```python
from build123d import *

# Parameters (mm, degrees)
SKETCH_1_W               = 130
SKETCH_1_H               = 180
EXTRUDE_1_DEPTH          = 400
SKETCH_2_R               = 37.5
CUT_EXTRUDE_1_DEPTH      = 458.493169348
CUT_EXTRUDE_START        = -350
CUT_EXTRUDE_2_DEPTH      = 350
PATTERN_CIRCULAR_1_COUNT = 4
MIRROR_START             = -350
MIRROR_1_COPY_1_DEPTH    = 350
MIRROR_1_COPY_2_DEPTH    = 350
MIRROR_1_COPY_3_DEPTH    = 350


with BuildPart() as part:
    # Sketch 1 → Extrude 1 (new body)
    with BuildSketch(Plane.XY):
        with Locations((-65, 90)):
            Rectangle(SKETCH_1_W, SKETCH_1_H)
    extrude(amount=EXTRUDE_1_DEPTH)

    # Sketch 2 → Cut-Extrude 1 (cut, through all)
    with BuildSketch(Plane.XY.offset(400)):
        with Locations((-65, 132.5)):
            Circle(SKETCH_2_R)
        with Locations((-65, 47.5)):
            Circle(SKETCH_2_R)
    extrude(amount=-CUT_EXTRUDE_1_DEPTH, mode=Mode.SUBTRACT)

    # Sketch 4 → Cut-Extrude 2 (cut)
    with BuildSketch(Plane(origin=(0, 0, 0), x_dir=(-1, 0, 0), z_dir=(0, 0, -1)).offset(CUT_EXTRUDE_START)):
        with BuildLine():
            Line((86.25, 169.306079661), (83.75, 164.975952642))
            ThreePointArc((83.75, 164.975952642), (91.516504294, 159.016504294), (97.475952642, 151.25))
            Line((97.475952642, 151.25), (101.806079661, 153.75))
            ThreePointArc((101.806079661, 153.75), (95.0520382, 162.5520382), (86.25, 169.306079661))
        make_face()
    cut_extrude_2 = extrude(amount=CUT_EXTRUDE_2_DEPTH, mode=Mode.SUBTRACT)

    # Pattern Circular 1: Cut-Extrude 2 ×4 about axis
    pattern_circular_1_axis = Axis((-65, 132.5, 0), (0, 0, 1))
    for i in range(1, PATTERN_CIRCULAR_1_COUNT):
        add(cut_extrude_2.rotate(pattern_circular_1_axis, i * 360 / PATTERN_CIRCULAR_1_COUNT), mode=Mode.SUBTRACT)

    # Mirror 1: Cut-Extrude 2 across plane
    add(cut_extrude_2.mirror(Plane.ZX.offset(90)), mode=Mode.SUBTRACT)

    # Mirror 1 copy 1 sketch → Mirror 1 copy 1 (cut)
    with BuildSketch(Plane(origin=(67.5, -17.5, 0), x_dir=(0, 1, 0), z_dir=(0, 0, -1)).offset(MIRROR_START)):
        with BuildLine():
            Line((86.25, -169.306079661), (83.75, -164.975952642))
            ThreePointArc((83.75, -164.975952642), (91.516504294, -159.016504294), (97.475952642, -151.25))
            Line((97.475952642, -151.25), (101.806079661, -153.75))
            ThreePointArc((101.806079661, -153.75), (95.0520382, -162.5520382), (86.25, -169.306079661))
        make_face()
    extrude(amount=MIRROR_1_COPY_1_DEPTH, mode=Mode.SUBTRACT)

    # Mirror 1 copy 2 sketch → Mirror 1 copy 2 (cut)
    with BuildSketch(Plane(origin=(-130, -85, 0), x_dir=(1, 0, 0), z_dir=(0, 0, -1)).offset(MIRROR_START)):
        with BuildLine():
            Line((86.25, -169.306079661), (83.75, -164.975952642))
            ThreePointArc((83.75, -164.975952642), (91.516504294, -159.016504294), (97.475952642, -151.25))
            Line((97.475952642, -151.25), (101.806079661, -153.75))
            ThreePointArc((101.806079661, -153.75), (95.0520382, -162.5520382), (86.25, -169.306079661))
        make_face()
    extrude(amount=MIRROR_1_COPY_2_DEPTH, mode=Mode.SUBTRACT)

    # Mirror 1 copy 3 sketch → Mirror 1 copy 3 (cut)
    with BuildSketch(Plane(origin=(-197.5, 112.5, 0), x_dir=(0, -1, 0), z_dir=(0, 0, -1)).offset(MIRROR_START)):
        with BuildLine():
            Line((86.25, -169.306079661), (83.75, -164.975952642))
            ThreePointArc((83.75, -164.975952642), (91.516504294, -159.016504294), (97.475952642, -151.25))
            Line((97.475952642, -151.25), (101.806079661, -153.75))
            ThreePointArc((101.806079661, -153.75), (95.0520382, -162.5520382), (86.25, -169.306079661))
        make_face()
    extrude(amount=MIRROR_1_COPY_3_DEPTH, mode=Mode.SUBTRACT)


solid = part.part
```
The listing builds one solid part. Answer for the finished solid, in the listing's coordinates (mm). A direction names the side the tool comes from. Coordinates: 2 decimals unless noted, no trailing zeros. Write each loop counter-clockwise with the first axis right and the second up, starting at its lowest first coordinate (ties: lowest second). Pieces come first, ordered by that corner, then holes. Notation, with made-up numbers: (60.25, -20.75) -> (88.25, -20.75) arc R30 ccw to (88.25, 18.25) -> close; hole circle Ø11 at (7.25, 57.5). An arc over 180 degrees is marked (long way). Write each question's results on one line, items separated by ' | '. Start each with the question number.
1) A cutting plane is placed at A-A (x = -65). Determine the outline of the cut face in (y, z), then the cut area to 3 significant figures.
2) A tool of negligible diameter and unlimited length cuts with its end or side. For faces 1 (the flat face through (-66, 91, 400)), 2 (the flat face through (-93, 76, 350)), from which of +Z, -Z, +X, -X, +Y, -Y can it reach the whole face along a straight path? Write none if from no direction.
3) A cutting plane is placed at C-C (z = 61.5). Count the separate pieces of the cut face and the enclosed holes in it, then the cut area to 3 significant figures.
4) Straight lines are drawn through the part: probe 1 along Y at (x, z) = (-65, 134.5); probe 2 along X at (y, z) = (132.5, 227); probe 3 along Y at (x, z) = (-80, 154.5). For each, find the intervals that lie inside material, in ascending order.
5) Flat-ended cylindrical pins translate along their axes: pin 1 Ø14.5 at (x, y) = (-90.5, 101) entering from -Z; pin 2 Ø5.5 at (x, y) = (-39, 18) entering from -Z. Find the tip coordinate at first contact, or state that the pin passes through.
6) A cutting plane is placed at B-B (y = 47.5). Determine the outline of the cut face in (x, z).
7) A cutting plane is placed at D-D (x = -92). Determine the outline of the cut face in (y, z).
8) For a pull along X with two mould halves and no side action, classify faces 3 (the flat face through (-66, 0, 197)), 4 (the cylindrical face through (-35.058, 17.338, 177.45)) as +X half, -X half, draft (parallel to the pull), parting line (faces both ways), or undercut.
Values follow:
1) outline: (0, 0) -> (10, 0) -> (10, 400) -> (0, 400) -> close; (85, 0) -> (95, 0) -> (95, 400) -> (85, 400) -> close; (170, 0) -> (180, 0) -> (180, 400) -> (170, 400) -> close | area: 12,000 mm²
2) face 1: +Z, +X, -X, +Y, -Y | face 2: -Z
3) separate pieces: 1 | enclosed holes: 2 | area: 13,700 mm²
4) probe 1: 0 to 10, 85 to 95, 170 to 180 | probe 2: -130 to -102.5, -27.5 to 0 | probe 3: 0 to 13.13, 81.87 to 98.13, 166.87 to 180
5) pin 1: z = 0 | pin 2: z = 350
6) outline: (-130, 0) -> (-102.5, 0) -> (-102.5, 400) -> (-130, 400) -> close; (-27.5, 0) -> (0, 0) -> (0, 400) -> (-27.5, 400) -> close
7) outline: (0, 0) -> (14.68, 0) -> (14.68, 350) -> (21.48, 350) -> (21.48, 400) -> (0, 400) -> close; (73.52, 350) -> (80.32, 350) -> (80.32, 0) -> (99.68, 0) -> (99.68, 350) -> (106.48, 350) -> (106.48, 400) -> (73.52, 400) -> close; (158.52, 350) -> (165.32, 350) -> (165.32, 0) -> (180, 0) -> (180, 400) -> (158.52, 400) -> close
8) face 3: draft | face 4: undercut
